```python
from build123d import *

# Parameters (mm, degrees)
CYLINDER_R        = 8
CYLINDER_DEPTH    = 10
CYLINDER001_R     = 12
CYLINDER001_DEPTH = 2
CYLINDER002_R     = 10
CYLINDER002_DEPTH = 8
FILLET_R          = 1


with BuildPart() as cylinder:
    # Cylinder → Cylinder (new body)
    with BuildSketch(Plane.XY):
        Circle(CYLINDER_R)
    extrude(amount=CYLINDER_DEPTH)


with BuildPart() as cylinder001:
    # Cylinder001 → Cylinder001 (new body)
    with BuildSketch(Plane.XY):
        Circle(CYLINDER001_R)
    extrude(amount=CYLINDER001_DEPTH)


with BuildPart() as fillet_body:
    # Cylinder002 → Cylinder002 (new body)
    with BuildSketch(Plane.XY.offset(2)):
        Circle(CYLINDER002_R)
    extrude(amount=CYLINDER002_DEPTH)

    # Fusion: union Cylinder001
    add(cylinder001.part)

    # Cut: cut Cylinder
    add(cylinder.part, mode=Mode.SUBTRACT)

    # Fillet
    fillet_edges = [fillet_body.edges().sort_by_distance(p)[0] for p in [
        (-12, 0, 0),
        (-8, 0, 0),
    ]]
    fillet(fillet_edges, radius=FILLET_R)


solid = fillet_body.part
```
Could you check a few things on this model? Use its own coordinates, in mm. A direction names the side the tool comes from. Coordinates: 2 decimals unless noted, no trailing zeros. Write each loop counter-clockwise with the first axis right and the second up, starting at its lowest first coordinate (ties: lowest second). Pieces come first, ordered by that corner, then holes. Notation, with made-up numbers: (72, 14.25) - (99, 14.25) arc R16 cw to (99, 24.25) - close; hole circle Ø9 at (21, 40.25). An arc over 180 degrees is marked (long way). Use a Markdown table: item, result.
Q1. Imagine slicing it at A-A (y = 0). List the corners of the cut face in (x, z) for me.
Geometry check:
| item | result |
|---|---|
| outline | (-12, 1) arc R1 ccw to (-11, 0) - (-9, 0) arc R1 ccw to (-8, 1) - (-8, 10) - (-10, 10) - (-10, 2) - (-12, 2) - close; (8, 1) arc R1 ccw to (9, 0) - (11, 0) arc R1 ccw to (12, 1) - (12, 2) - (10, 2) - (10, 10) - (8, 10) - close |
Q2. Which directions (+Z, -Z, +X, -X, +Y, -Y) give clear straight access to the entire face, cutting with the end or side of a thin tool? Please do faces 1 (the flat face through (0, 8.2, 10)), 2 (the flat face through (-5, 9, 2)).
Geometry check:
| item | result |
|---|---|
| face 1 | +Z, +X, -X, +Y, -Y |
| face 2 | +Z |
Q3. Imagine slicing it at C-C (z = 5.5). List the corners of the cut face in (x, y) for me, and give its area (3 significant figures).
Geometry check:
| item | result |
|---|---|
| outline | circle Ø20 at (0, 0); hole circle Ø16 at (0, 0) |
| area | 113 mm2 |
Q4. Thinking about a two-plate mould opening in Y: for faces 3 (the cylindrical face through (-2.17, -9.76, 5.94)), 4 (the cylindrical face through (-1.73, -7.81, 5.44)), 5 (the flat face through (2, -9, 0)), which applies, +Y half, -Y half, draft (parallel to the pull), parting line (faces both ways), or undercut?
Geometry check:
| item | result |
|---|---|
| face 3 | parting line |
| face 4 | undercut |
| face 5 | draft |
Q5. I'm going to push flat-ended pins straight in: pin 1 Ø1 at (x, z) = (5, 6.5) entering from +Y; pin 2 Ø1.5 at (x, z) = (2, 8.5) entering from -Y; pin 3 Ø1.5 at (y, z) = (3.5, 3) entering from -X. Where does each tip first touch, or does it pass through?
Geometry check:
| item | result |
|---|---|
| pin 1 | stops at y = 8.93 |
| pin 2 | stops at y = -9.92 |
| pin 3 | stops at x = -9.61 |
Q6. Please list where these lines run through material, in increasing order: L1, parallel to Y at x = 0, z = 6.5; L2, parallel to Y at x = 7, z = 7.75; L3, parallel to Z at x = 10, y = -3.5.
Geometry check:
| item | result |
|---|---|
| L1 | y = -10 to -8, 8 to 10 |
| L2 | y = -7.14 to -3.87, 3.87 to 7.14 |
| L3 | z = 0 to 2 |
